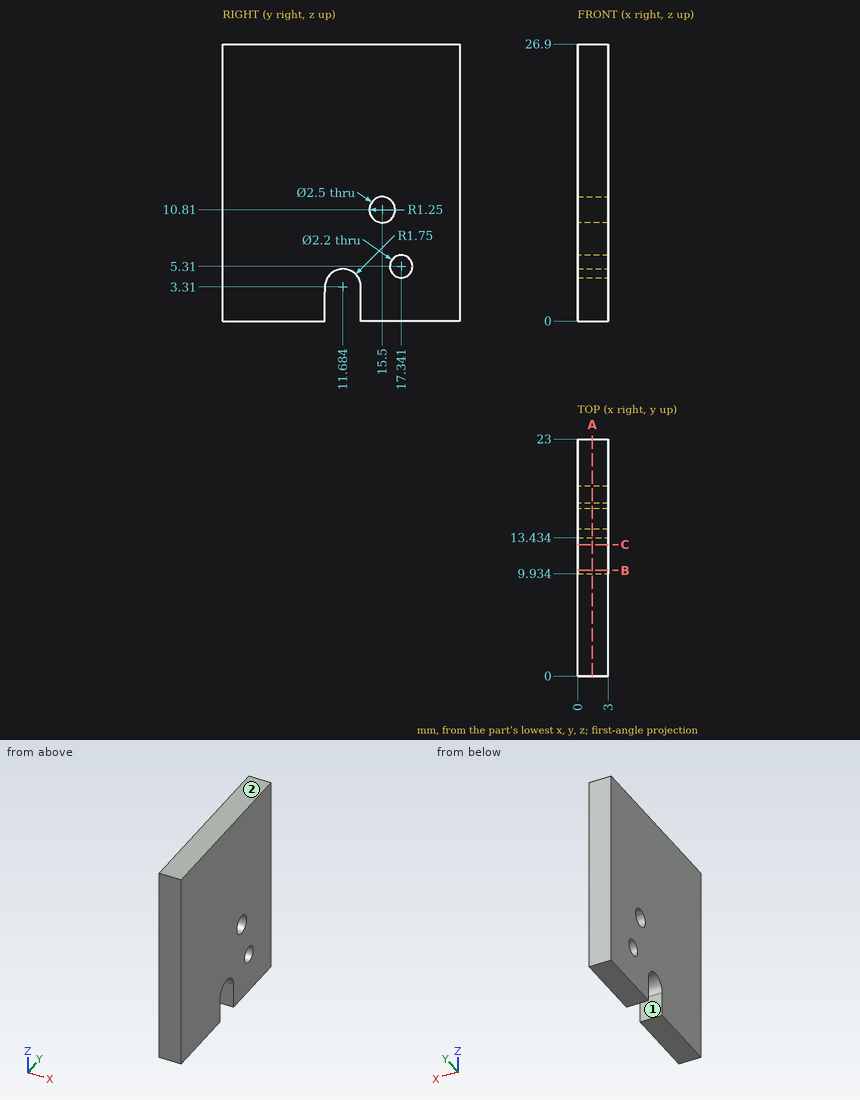
Could you check a few things on this drawing? It's one solid part, dimensions in mm from its lowest x, y, z. A direction names the side the tool comes from. Round coordinates to 2 decimals unless told otherwise and drop trailing zeros. Loops run counter-clockwise (first coordinate to the right, second up) from the corner with the lowest first, then second, coordinate; pieces in that order, holes last. Notation, with made-up numbers: (81, 14) -> (106, 14) arc R15 ccw to (106, 30) -> close; hole circle Ø7 at (40.5, 42). An arc over 180 degrees is marked (long way). Answer as CSV lines item,"result".
1. For pin 1 (2 mm diameter, centred on y = 15.5, z = 10.81, fed in from +X); pin 2 (6 mm diameter, centred on y = 2.5, z = 21.5, fed in from -X), each with a flat end and sliding along its axis, tell me the tip position at first contact or that it passes through.
Final values:
pin 1,"passes through"
pin 2,"stops at x = 0"
2. If we section it at B-B on y = 10.25: Please give me the cut outline in (x, z).
Final values:
outline,"(0, 4.31) -> (3, 4.31) -> (3, 26.9) -> (0, 26.9) -> close"
3. If we section it at A-A on x = 1.45: Count the separate pieces of the cut face and the enclosed holes in it, plus the area to 3 significant figures.
Final values:
separate pieces,"1"
enclosed holes,"2"
area,"594 mm^2"
4. Which directions (+Z, -Z, +X, -X, +Y, -Y) give clear straight access to the entire face, cutting with the end or side of a thin tool? Please do the marked faces 1 and 2.
Final values:
face 1,"-Z, +X, -X"
face 2,"+Z, +X, -X, +Y, -Y"
5. If I drill on L1, parallel to Y at x = 2.45, z = 1.25 (1 decimal); L2, parallel to Z at x = 1.75, y = 15.5; L3, parallel to Z at x = 1.75, y = 15.75 (1 decimal), over which ranges is the centre line in solid material (lowest first)?
Final values:
L1,"y = 0 to 9.9, 13.4 to 23"
L2,"z = 0 to 9.56, 12.06 to 26.9"
L3,"z = 0 to 9.6, 12 to 26.9"
6. If we section it at C-C on y = 12.75: Please give me the cut outline in (x, z).
Final values:
outline,"(0, 4.7) -> (3, 4.7) -> (3, 26.9) -> (0, 26.9) -> close"
